```python
from build123d import *

# Parameters (mm, degrees)
SKETCH1_W           = 1219.2
SKETCH1_H           = 1771.65
BOSS_EXTRUDE1_DEPTH = 19.05
SKETCH3_W           = 508
SKETCH3_H           = 685.8
CUT_EXTRUDE2_DEPTH  = 20.05
SKETCH5_W           = 846.4296
SKETCH5_H           = 758.825
CUT_EXTRUDE4_DEPTH  = 20.05
CUT_EXTRUDE12_DEPTH = 846.4296
CUT_EXTRUDE5_DEPTH  = 12.7
CUT_EXTRUDE6_DEPTH  = 7.35
CUT_EXTRUDE11_DEPTH = 12.7
CUT_EXTRUDE8_DEPTH  = 1772.65
CUT_EXTRUDE10_DEPTH = 1220.2
CHAMFER2_SIZE       = 2.032


with BuildPart() as part:
    # Sketch1 → Boss-Extrude1 (new body)
    with BuildSketch(Plane(origin=(0, 0, 0), x_dir=(1, 0, 0), z_dir=(0, 1, 0))):
        with Locations((609.6, 885.825)):
            Rectangle(SKETCH1_W, SKETCH1_H)
    extrude(amount=-BOSS_EXTRUDE1_DEPTH)

    # Sketch3 → Cut-Extrude2 (cut, through all)
    with BuildSketch(Plane(origin=(0, 0, 0), x_dir=(1, 0, 0), z_dir=(0, 1, 0))):
        with Locations((1046.1625, 342.9)):
            Rectangle(SKETCH3_W, SKETCH3_H)
    extrude(amount=-CUT_EXTRUDE2_DEPTH, mode=Mode.SUBTRACT)

    # Sketch5 → Cut-Extrude4 (cut, through all)
    with BuildSketch(Plane(origin=(0, 0, 0), x_dir=(1, 0, 0), z_dir=(0, 1, 0))):
        with Locations((722.3252, 1392.2375)):
            Rectangle(SKETCH5_W, SKETCH5_H)
    extrude(amount=-CUT_EXTRUDE4_DEPTH, mode=Mode.SUBTRACT)

    # Sketch18 → Cut-Extrude12 (cut)
    with BuildSketch(Plane(origin=(299.1104, 0, 0), x_dir=(0, 0, -1), z_dir=(1, 0, 0))):
        with BuildLine():
            Line((1009.601754844, -19.05), (1771.65, -19.05))
            Line((1771.65, -19.05), (1771.65, 0))
            Line((1771.65, 0), (1014.82750315, 0))
            ThreePointArc((1014.82750315, 0), (1012.106135013, -9.495238202), (1009.601754844, -19.05))
        make_face()
    extrude(amount=CUT_EXTRUDE12_DEPTH, mode=Mode.SUBTRACT)

    # Sketch7 → Cut-Extrude5 (cut)
    with BuildSketch(Plane(origin=(0, 0, 0), x_dir=(1, 0, 0), z_dir=(0, 1, 0))):
        with BuildLine():
            Line((281.3685, 717.55), (478.2185, 717.55))
            ThreePointArc((478.2185, 717.55), (491.688884182, 711.970384182), (497.2685, 698.5))
            Line((497.2685, 698.5), (497.2685, 438.15))
            ThreePointArc((497.2685, 438.15), (491.688884182, 424.679615818), (478.2185, 419.1))
            Line((478.2185, 419.1), (281.3685, 419.1))
            ThreePointArc((281.3685, 419.1), (267.898115818, 424.679615818), (262.3185, 438.15))
            Line((262.3185, 438.15), (262.3185, 698.5))
            ThreePointArc((262.3185, 698.5), (267.898115818, 711.970384182), (281.3685, 717.55))
        make_face()
    extrude(amount=-CUT_EXTRUDE5_DEPTH, mode=Mode.SUBTRACT)

    # Sketch8 → Cut-Extrude6 (cut, through all)
    with BuildSketch(Plane(origin=(0, -12.7, 0), x_dir=(1, 0, 0), z_dir=(0, 1, 0))):
        Polygon((294.0685, 704.85), (275.0185, 685.8), (275.0185, 450.85), (294.0685, 431.8), (465.5185, 431.8), (484.5685, 450.85), (484.5685, 685.8), (465.5185, 704.85), align=None)
    extrude(amount=-CUT_EXTRUDE6_DEPTH, mode=Mode.SUBTRACT)

    # Sketch17 → Cut-Extrude11 (cut)
    with BuildSketch(Plane(origin=(0, 0, 0), x_dir=(1, 0, 0), z_dir=(0, 1, 0))):
        with BuildLine():
            Line((389.412860427, 806.45), (673.130860427, 806.45))
            ThreePointArc((673.130860427, 806.45), (695.355860427, 784.225), (673.130860427, 762))
            Line((673.130860427, 762), (389.412860427, 762))
            ThreePointArc((389.412860427, 762), (367.187860427, 784.225), (389.412860427, 806.45))
        make_face()
        with BuildLine():
            Line((389.412860427, 330.2), (673.130860427, 330.2))
            ThreePointArc((673.130860427, 330.2), (695.355860427, 352.425), (673.130860427, 374.65))
            Line((673.130860427, 374.65), (389.412860427, 374.65))
            ThreePointArc((389.412860427, 374.65), (367.187860427, 352.425), (389.412860427, 330.2))
        make_face()
    extrude(amount=-CUT_EXTRUDE11_DEPTH, mode=Mode.SUBTRACT)

    # Sketch12 → Cut-Extrude8 (cut, through all)
    with BuildSketch(Plane.XY):
        Polygon((209.2579, 0), (190.2079, 0), (190.2079, -6.096), (187.7949, -6.096), (187.7949, -9.525), (211.6709, -9.525), (211.6709, -6.096), (209.2579, -6.096), align=None)
        Polygon((237.4519, 0), (230.0859, 0), (230.0859, -2.54), (228.0539, -2.54), (228.0539, -9.525), (239.4839, -9.525), (239.4839, -2.54), (237.4519, -2.54), align=None)
    extrude(amount=-CUT_EXTRUDE8_DEPTH, mode=Mode.SUBTRACT)

    # Sketch16 → Cut-Extrude10 (cut, through all)
    with BuildSketch(Plane.ZY):
        Polygon((-1438.8084, -9.525), (-1414.4244, -9.525), (-1414.4244, -5.969), (-1417.0914, -5.969), (-1417.0914, 0), (-1436.1414, 0), (-1436.1414, -5.969), (-1438.8084, -5.969), align=None)
    extrude(amount=-CUT_EXTRUDE10_DEPTH, mode=Mode.SUBTRACT)

    # Chamfer2
    chamfer2_edges = [part.edges().sort_by_distance(p)[0] for p in [
        (367.187860427, 0, -784.225),
        (531.271860427, 0, -762),
        (695.355860427, 0, -784.225),
        (531.271860427, 0, -806.45),
        (367.187860427, 0, -352.425),
        (531.271860427, 0, -330.2),
        (695.355860427, 0, -352.425),
        (531.271860427, 0, -374.65),
        (1005.68125, 0, -685.8),
        (219.6719, 0, -1771.65),
        (95.10395, 0, -1771.65),
        (219.6719, 0, 0),
        (514.8072, 0, 0),
        (792.1625, 0, -342.9),
        (1145.54, 0, -1603.8957),
        (299.1104, 0, -1214.9582),
        (0, 0, -708.5457),
        (268.28115, 0, -1771.65),
        (299.1104, 0, -1603.8957),
        (722.3252, 0, -1012.825),
        (1145.54, 0, -1214.9582),
        (0, 0, -1603.8957),
        (1182.37, 0, -1771.65),
        (95.10395, 0, 0),
        (491.688884182, 0, -424.679615818),
        (497.2685, 0, -568.325),
        (491.688884182, 0, -711.970384182),
        (379.7935, 0, -717.55),
        (267.898115818, 0, -711.970384182),
        (262.3185, 0, -568.325),
        (267.898115818, 0, -424.679615818),
        (379.7935, 0, -419.1),
    ]]
    chamfer(chamfer2_edges, length=CHAMFER2_SIZE)


solid = part.part
```
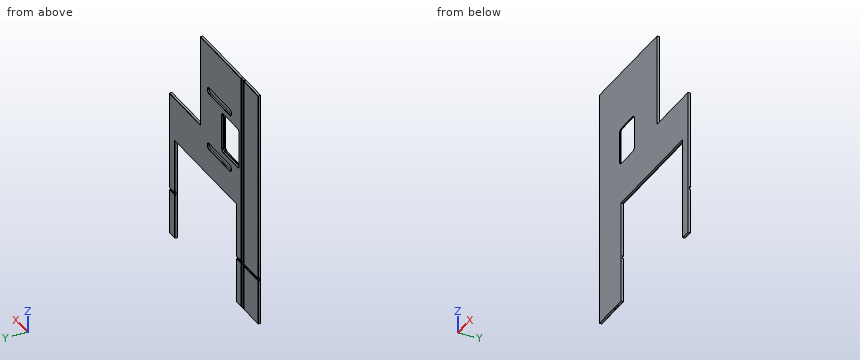
Geometry: final body of the model. Coordinates: model frame, mm. Round coordinates to 2 decimals unless told otherwise and drop trailing zeros. Order: outer loops, then holes, each group sorted by start corner. A loop starts at its lowest first (then second) coordinate and runs counter-clockwise, first axis right, second up. Notation, with made-up numbers: (49, 73) - (81, 73) arc R31 ccw to (81, 105) - close; hole circle Ø5 at (24.25, -19.5). An arc over 180 degrees is marked (long way). Use CSV: the item, a comma, the result in double quotes. Start each with the question number.
Q1. Material intervals for line 1 along X through (y, z) = (-2.5, -299); line 2 along X through (y, z) = (-8.5, -1676.5); line 3 along X through (y, z) = (-3.75, -175), sorted ascending. Write a range as from..to.
Q2. Section query B-B (z = -1633). Return loops of the section in (x, y) (3 decimals), and give its area (3 significant figures).
Q3. Section query C-C (x = 524). Return loops of the section in (y, z) (3 decimals).
Q4. First-contact query: pin 1 (1 mm diameter, centred on x = 783.5, y = -4, fed in from -Z) (3 decimals); pin 2 (5 mm diameter, centred on x = 1170, y = -2, fed in from +Z). Flat tips, straight axial feed; report the tip coordinate or a pass-through.
Q5. Section query A-A (x = 330.5). Return loops of the section in (y, z) (3 decimals), and give its area (3 significant figures).
Result set:
1,line 1,"x = 0..190.21, 209.26..230.09, 237.45..792.16"
1,line 2,"x = 0..187.79, 211.67..228.05, 239.48..299.11, 1145.54..1219.2"
1,line 3,"x = 0..190.21, 209.26..228.05, 239.48..792.16"
2,outline,"(0, -19.05) - (299.11, -19.05) - (299.11, -2.032) - (297.078, 0) - (237.452, 0) - (237.452, -2.54) - (239.484, -2.54) - (239.484, -9.525) - (228.054, -9.525) - (228.054, -2.54) - (230.086, -2.54) - (230.086, 0) - (209.258, 0) - (209.258, -6.096) - (211.671, -6.096) - (211.671, -9.525) - (187.795, -9.525) - (187.795, -6.096) - (190.208, -6.096) - (190.208, 0) - (2.032, 0) - (0, -2.032) - close; (1145.54, -19.05) - (1219.2, -19.05) - (1219.2, 0) - (1147.572, 0) - (1145.54, -2.032) - close"
2,area,"6,800 mm2"
3,outline,"(-19.05, -1009.602) arc R433.616 cw to (-6.906, -1012.825) - (-2.032, -1012.825) - (0, -1010.793) - (0, -808.482) - (-2.032, -806.45) - (-12.7, -806.45) - (-12.7, -762) - (-2.032, -762) - (0, -759.968) - (0, -376.682) - (-2.032, -374.65) - (-12.7, -374.65) - (-12.7, -330.2) - (-2.032, -330.2) - (0, -328.168) - (0, -2.032) - (-2.032, 0) - (-19.05, 0) - close"
4,pin 1,"stops at z = -1012.825"
4,pin 2,"stops at z = -685.8"
5,outline,"(-19.05, -1009.602) arc R433.616 cw to (-6.906, -1012.825) - (-2.032, -1012.825) - (0, -1010.793) - (0, -719.582) - (-2.032, -717.55) - (-12.7, -717.55) - (-12.7, -704.85) - (-19.05, -704.85) - close; (-19.05, -431.8) - (-12.7, -431.8) - (-12.7, -419.1) - (-2.032, -419.1) - (0, -417.068) - (0, -2.032) - (-2.032, 0) - (-19.05, 0) - close"
5,area,"13,700 mm2"
